Verification items for the finished model (mm, model axes). A direction names the side the tool comes from. Coordinates: 2 decimals unless noted, no trailing zeros. Order: outer loops, then holes, each group sorted by start corner. A loop starts at its lowest first (then second) coordinate and runs counter-clockwise, first axis right, second up.
Q1. Cross-section at A-A, the plane y = 6.5. Record the boundary of the cut face in (x, z), and give its area (3 significant figures).
Q2. Thickness scan on line 1 (Z direction, x = 14, y = 11); line 2 (X direction, y = 9, z = 18); line 3 (Z direction, x = -10, y = 11.75). Record the ranges inside material, lowest first.
Q3. Cross-section at B-B, the plane x = -17. Record the boundary of the cut face in (y, z), and give its area (3 significant figures).
Q4. Draft check along X on faces 1 (the cylindrical face through (-21.685, 4.902, -13.671)), 2 (the cylindrical face through (-34.245, 4.902, -23.045)), 3 (the flat face through (0, 12, -18)). Enter one of: pulls with the +X half, pulls with the -X half, needs draft (parallel to the pull), parting line crosses it, or undercut.
Q5. Cross-section at D-D, the plane z = 1.5. Record the boundary of the cut face in (x, y), and give its area (3 significant figures).
Q6. Depth check by flat-ended pin: P1, Ø1.5, axis at x = -12, y = 10.5, coming from the -Z side; P2, Ø1.5, axis at x = -18, y = 8, coming from the +Z side; P3, Ø8, axis at x = 11, y = 2.5, coming from the +Z side. Enter the tip coordinate at first touch or a pass-through.
Q7. Cross-section at C-C, the plane z = -24. Record the boundary of the cut face in (x, y), and give its area (3 significant figures).
Q8. Set-up check for faces 4 (the cylindrical face through (16.77, 4.9, 0.45)), 5 (the cylindrical face through (-16.54, 4.902, 0.556)), 6 (the flat face through (-1.573, 4.902, 28.272)), 7 (the flat face through (-6.26, 4.9, 11.43)), 8 (the cylindrical face through (0.217, 4.902, -50.076)): record each of +Z, -Z, +X, -X, +Y, -Y from which the full face is reachable in a straight line by a thin tool's end or side.
from build123d import *

# Parameters (mm, degrees)
SKETCH_1_R      = 6.5
EXTRUDE_3_DEPTH = 10
SCALE_1_SCALE   = 1.4


with BuildPart() as part:
    # 草图1 → 凸台-拉伸3 (new body)
    # profile 1 of 12: a face of its own
    with BuildSketch(Plane(origin=(0, 0, 0), x_dir=(1, 0, 0), z_dir=(0, 1, 0))):
        with BuildLine():
            ThreePointArc((5.859785995, 33.829217687), (7.388132252, 34.23249014), (8.953138838, 34.454357972))
            ThreePointArc((8.953138838, 34.454357972), (0, 40), (-8.953138838, 34.454357972))
            ThreePointArc((-8.953138838, 34.454357972), (-7.388132252, 34.23249014), (-5.859785995, 33.829217687))
            ThreePointArc((-5.859785995, 33.829217687), (0, 37), (5.859785995, 33.829217687))
        make_face()
    # profile 2 of 12: a face of its own
    with BuildSketch(Plane(origin=(0, 0, 0), x_dir=(1, 0, 0), z_dir=(0, 1, 0))):
        with BuildLine():
            ThreePointArc((0, 30), (7.005568982, 34.149386276), (15.123058987, 33.515541466))
            ThreePointArc((15.123058987, 33.515541466), (24.442500681, 20.921509808), (17.460562256, 6.896027189))
            ThreePointArc((17.460562256, 6.896027189), (11.894938122, 3.870741491), (6, 1.551640353))
            Line((6, 1.551640353), (0, -20))
            Line((0, -20), (-6, 1.551640353))
            ThreePointArc((-6, 1.551640353), (-11.894938122, 3.870741491), (-17.460562256, 6.896027189))
            ThreePointArc((-17.460562256, 6.896027189), (-24.442500681, 20.921509808), (-15.123058987, 33.515541466))
            ThreePointArc((-15.123058987, 33.515541466), (-7.005568982, 34.149386276), (0, 30))
        make_face()
        with Locations(Location((-13, 20, 0), (0, 0, 270))):
            Circle(SKETCH_1_R, mode=Mode.SUBTRACT)
        with Locations(Location((13, 20, 0), (0, 0, 270))):
            Circle(SKETCH_1_R, mode=Mode.SUBTRACT)
    # profile 3 of 12: a face of its own
    with BuildSketch(Plane(origin=(0, 0, 0), x_dir=(1, 0, 0), z_dir=(0, 1, 0))):
        with BuildLine():
            ThreePointArc((-1.7, -7), (-7.439120142, -11.25), (-13.178240283, -7))
            ThreePointArc((-13.178240283, -7), (-7.439120142, -14.75), (-1.7, -7))
        make_face()
    # profile 4 of 12: a face of its own
    with BuildSketch(Plane(origin=(0, 0, 0), x_dir=(1, 0, 0), z_dir=(0, 1, 0))):
        with BuildLine():
            ThreePointArc((1.7, -7), (7.439120142, -14.75), (13.178240283, -7))
            ThreePointArc((13.178240283, -7), (7.439120142, -11.25), (1.7, -7))
        make_face()
    # profile 5 of 12: a face of its own
    with BuildSketch(Plane(origin=(0, 0, 0), x_dir=(1, 0, 0), z_dir=(0, 1, 0))):
        with BuildLine():
            ThreePointArc((1.7, -7), (1.48214902, -9.46728311), (2.279456101, -11.812330319))
            Line((2.279456101, -11.812330319), (2.986703917, -9.271938557))
            ThreePointArc((2.986703917, -9.271938557), (2.218269676, -8.206809162), (1.7, -7))
        make_face()
    # profile 6 of 12: a face of its own
    with BuildSketch(Plane(origin=(0, 0, 0), x_dir=(1, 0, 0), z_dir=(0, 1, 0))):
        with BuildLine():
            Line((2.986703917, -9.271938557), (2.279456101, -11.812330319))
            ThreePointArc((2.279456101, -11.812330319), (9.862665709, -14.238754584), (13.178240283, -7))
            ThreePointArc((13.178240283, -7), (8.744619259, -11.106250682), (2.986703917, -9.271938557))
        make_face()
    # profile 7 of 12: a face of its own
    with BuildSketch(Plane(origin=(0, 0, 0), x_dir=(1, 0, 0), z_dir=(0, 1, 0))):
        with BuildLine():
            ThreePointArc((1.7, -7), (1.48214902, -9.46728311), (2.279456101, -11.812330319))
            Line((2.279456101, -11.812330319), (2.986703917, -9.271938557))
            ThreePointArc((2.986703917, -9.271938557), (2.218269676, -8.206809162), (1.7, -7))
        make_face()
    # profile 8 of 12: a face of its own
    with BuildSketch(Plane(origin=(0, 0, 0), x_dir=(1, 0, 0), z_dir=(0, 1, 0))):
        with BuildLine():
            Line((2.986703917, -9.271938557), (2.279456101, -11.812330319))
            ThreePointArc((2.279456101, -11.812330319), (9.862665709, -14.238754584), (13.178240283, -7))
            ThreePointArc((13.178240283, -7), (8.744619259, -11.106250682), (2.986703917, -9.271938557))
        make_face()
    # profile 9 of 12: a face of its own
    with BuildSketch(Plane(origin=(0, 0, 0), x_dir=(1, 0, 0), z_dir=(0, 1, 0))):
        with BuildLine():
            ThreePointArc((-13.178240283, -7), (-9.862665709, -14.238754584), (-2.279456101, -11.812330319))
            Line((-2.279456101, -11.812330319), (-2.986703917, -9.271938557))
            ThreePointArc((-2.986703917, -9.271938557), (-8.744619259, -11.106250682), (-13.178240283, -7))
        make_face()
    # profile 10 of 12: a face of its own
    with BuildSketch(Plane(origin=(0, 0, 0), x_dir=(1, 0, 0), z_dir=(0, 1, 0))):
        with BuildLine():
            Line((-2.986703917, -9.271938557), (-2.279456101, -11.812330319))
            ThreePointArc((-2.279456101, -11.812330319), (-1.48214902, -9.46728311), (-1.7, -7))
            ThreePointArc((-1.7, -7), (-2.218269676, -8.206809162), (-2.986703917, -9.271938557))
        make_face()
    # profile 11 of 12: a face of its own
    with BuildSketch(Plane(origin=(0, 0, 0), x_dir=(1, 0, 0), z_dir=(0, 1, 0))):
        with BuildLine():
            ThreePointArc((-13.178240283, -7), (-9.862665709, -14.238754584), (-2.279456101, -11.812330319))
            Line((-2.279456101, -11.812330319), (-2.986703917, -9.271938557))
            ThreePointArc((-2.986703917, -9.271938557), (-8.744619259, -11.106250682), (-13.178240283, -7))
        make_face()
    # profile 12 of 12: a face of its own
    with BuildSketch(Plane(origin=(0, 0, 0), x_dir=(1, 0, 0), z_dir=(0, 1, 0))):
        with BuildLine():
            Line((-2.986703917, -9.271938557), (-2.279456101, -11.812330319))
            ThreePointArc((-2.279456101, -11.812330319), (-1.48214902, -9.46728311), (-1.7, -7))
            ThreePointArc((-1.7, -7), (-2.218269676, -8.206809162), (-2.986703917, -9.271938557))
        make_face()
    extrude(amount=EXTRUDE_3_DEPTH)


with BuildPart() as part_1:
    # 缩放比例1: scaled about (0, 5, -14.807027766)
    add(part.part.scale(SCALE_1_SCALE).moved(Location((0, -2, 5.922811106))))


solid = part_1.part
Check values:
1. outline: (-24.44, -3.73) arc R21 ccw to (-21.17, -41) arc R18.9 ccw to (-12.53, -42.31) arc R14 ccw to (12.53, -42.31) arc R18.9 ccw to (21.17, -41) arc R21 ccw to (24.44, -3.73) arc R72.1 ccw to (8.4, 3.75) - (4.18, 18.9) arc R8.4 cw to (18.45, 15.72) arc R8.4 ccw to (3.19, 22.46) - (0, 33.92) - (-3.19, 22.46) arc R8.4 ccw to (-18.45, 15.72) arc R8.4 cw to (-4.18, 18.9) - (-8.4, 3.75) arc R72.1 ccw to start; hole circle Ø18.2 at (-18.2, -22.08); hole (-8.2, -41.44) arc R9.8 ccw to (8.2, -41.44) arc R18.9 cw to (0, -36.08) arc R18.9 cw to start; hole circle Ø18.2 at (18.2, -22.08)
1. area: 2,550 mm2
2. line 1: z = -42.38 to -30.15, -14 to 1.68, 20.87 to 25.77
2. line 2: x = -18.81 to -17.36, -4.43 to 4.43, 17.36 to 18.81
2. line 3: z = -45.88 to -26.02, -18.13 to 3.21, 21.66 to 26.56
3. outline: (-2, -42.15) - (12, -42.15) - (12, -31.1) - (-2, -31.1) - close; (-2, -13.06) - (12, -13.06) - (12, 0.34) - (-2, 0.34) - close; (-2, 18.49) - (12, 18.49) - (12, 23.39) - (-2, 23.39) - close
3. area: 411 mm2
4. face 1: undercut
4. face 2: pulls with the -X half
4. face 3: needs draft
5. outline: (-14.42, -2) - (14.42, -2) - (14.42, 12) - (-14.42, 12) - close
5. area: 404 mm2
6. P1: stops at z = -44.41
6. P2: stops at z = 23.06
6. P3: stops at z = 26.57
7. outline: (-34.15, -2) - (-27.09, -2) - (-27.09, 12) - (-34.15, 12) - close; (-9.31, -2) - (9.31, -2) - (9.31, 12) - (-9.31, 12) - close; (27.09, -2) - (34.15, -2) - (34.15, 12) - (27.09, 12) - close
7. area: 458 mm2
8. face 4: +X, +Y, -Y
8. face 5: -X, +Y, -Y
8. face 6: +Z, +Y, -Y
8. face 7: +Y, -Y
8. face 8: -Z, +Y, -Y
